Can you work these out from the drawing? Everything is in mm from the part's minimum corner. A direction names the side the tool comes from. Round coordinates to 2 decimals unless told otherwise and drop trailing zeros. Write each loop counter-clockwise with the first axis right and the second up, starting at its lowest first coordinate (ties: lowest second). Pieces come first, ordered by that corner, then holes. Notation, with made-up numbers: (20.5, -22) -> (42.5, -22) arc R36 ccw to (42.5, 13) -> close; hole circle Ø5 at (40.5, 25). An arc over 180 degrees is marked (long way). One line per question, with ' | ' between items. Start each with the question number.
1. For pin 1 Ø12 at (y, z) = (29.5, 19.5) entering from +X; pin 2 Ø6 at (x, z) = (14.5, 25) entering from -Y; pin 3 Ø1.9 at (x, y) = (25, 27.5) entering from +Z; pin 4 Ø3 at (x, y) = (4, 24) entering from +Z, each with a flat end and sliding along its axis, tell me the tip position at first contact or that it passes through.
2. Imagine slicing it at B-B, the plane y = 23.5. List the corners of the cut face in (x, z) for me, and give its area (3 significant figures).
3. For the marked faces 1, 2 and 3, which set-ups out of +Z, -Z, +X, -X, +Y, -Y let a thin tool reach every point of the face, with its end or its side?
4. If I drill on line 1 along Y through (x, z) = (5, 1) (1 decimal); line 2 along Z through (x, y) = (21, 21); line 3 along X through (y, z) = (31.5, 34.5), over which ranges is the centre line in solid material (lowest first)? Write a range as [from, to].
5. Imagine slicing it at C-C, the plane y = 27.5. List the corners of the cut face in (x, z) for me (1 decimal), and give its area (3 significant figures).
6. Imagine slicing it at A-A, the plane x = 16. List the corners of the cut face in (y, z) for me.
7. Imagine slicing it at D-D, the plane x = 5. List the corners of the cut face in (y, z) for me (1 decimal).
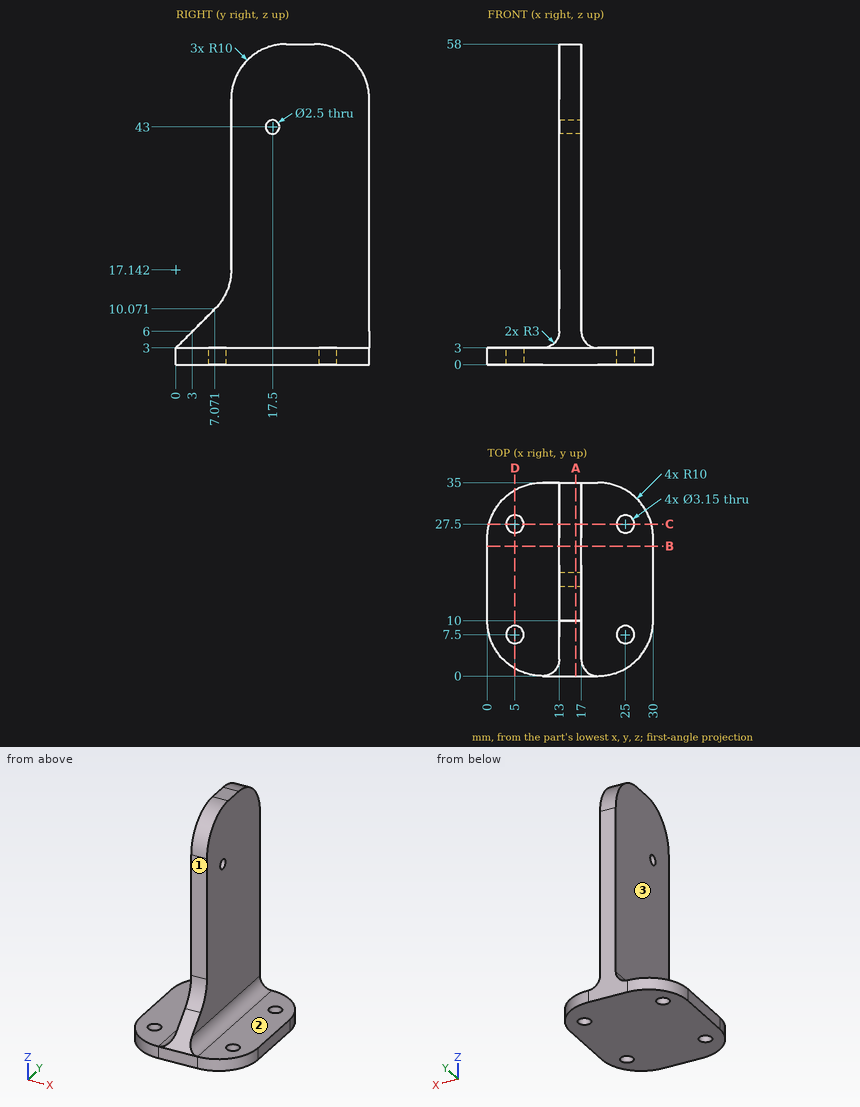
Geometry results:
1) pin 1: stops at x = 17 | pin 2: stops at y = 10 | pin 3: passes through | pin 4: stops at z = 3
2) outline: (0, 0) -> (30, 0) -> (30, 3) -> (20, 3) arc R3 cw to (17, 6) -> (17, 58) -> (13, 58) -> (13, 6) arc R3 cw to (10, 3) -> (0, 3) -> close | area: 314 mm2
3) face 1: +Z, +X, -X, -Y | face 2: +Z, +X, +Y, -Y | face 3: +Z, -X, +Y, -Y
4) line 1: y = [1.3, 5.9], [9.1, 25.9], [29.1, 33.7] | line 2: z = [0, 3] | line 3: x = [13, 17]
5) outline: (0.3, 0) -> (3.4, 0) -> (3.4, 3) -> (0.3, 3) -> close; (6.6, 0) -> (23.4, 0) -> (23.4, 3) -> (20, 3) arc R3 cw to (17, 6) -> (17, 57.7) -> (13, 57.7) -> (13, 6) arc R3 cw to (10, 3) -> (6.6, 3) -> close; (26.6, 0) -> (29.7, 0) -> (29.7, 3) -> (26.6, 3) -> close | area: 292 mm2
6) outline: (0, 0) -> (35, 0) -> (35, 48) arc R10 ccw to (25, 58) -> (20, 58) arc R10 ccw to (10, 48) -> (10, 17.14) arc R10 cw to (7.07, 10.07) -> (0, 3) -> close; hole circle Ø2.5 at (17.5, 43)
7) outline: (1.3, 0) -> (5.9, 0) -> (5.9, 3) -> (1.3, 3) -> close; (9.1, 0) -> (25.9, 0) -> (25.9, 3) -> (9.1, 3) -> close; (29.1, 0) -> (33.7, 0) -> (33.7, 3) -> (29.1, 3) -> close
